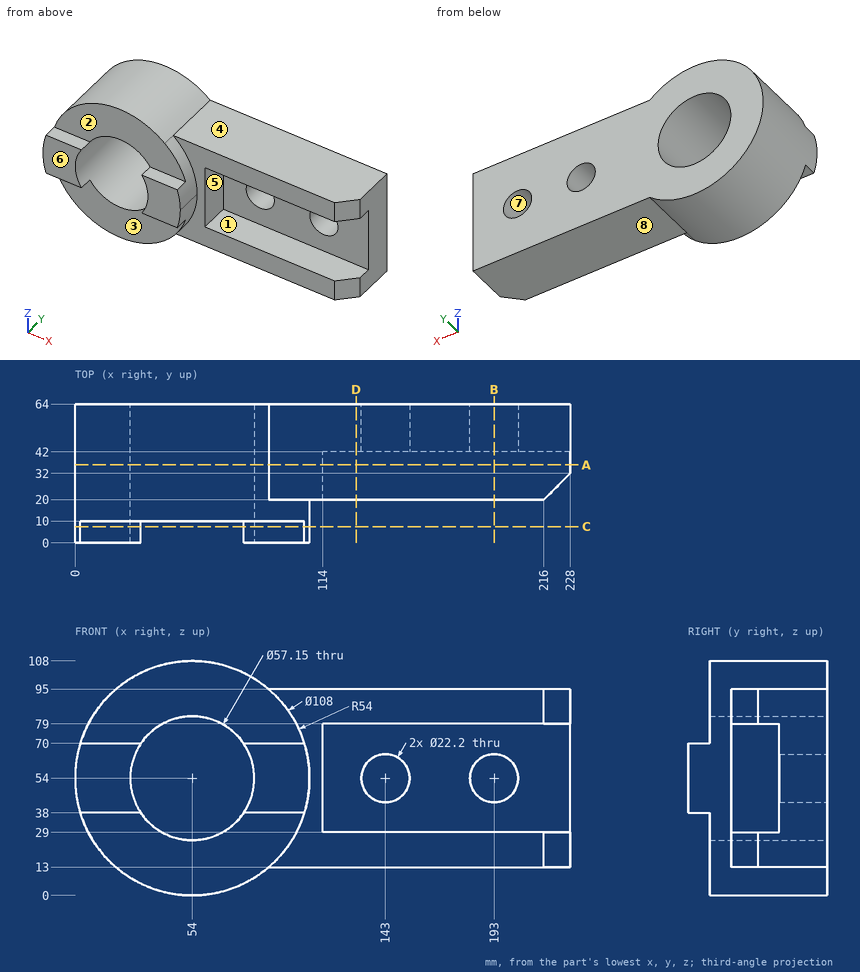
For this review, use the dimensioned drawing (mm, ordinates from the lowest corner) and the shaded views. A direction names the side the tool comes from. Give positions to 0.01 mm unless a question says otherwise; leave off trailing zeros. Loops run counter-clockwise (first coordinate to the right, second up) from the corner with the lowest first, then second, coordinate; pieces in that order, holes last.
Item 1: Take a section at D-D, the plane x = 129.5. State the section outline as (y, z) points.
Item 2: For line 1 along Z through (x, y) = (160, 33.5); line 2 along X through (y, z) = (54, 54) (3 decimals); line 3 along Z through (x, y) = (193, 47), list the stretches that pass through material, from the lowest coordinate up.
Item 3: Tool access review of the marked faces 1, 2, 3 and 4: name each direction out of +Z, -Z, +X, -X, +Y, -Y from which nothing blocks a thin tool from reaching the whole face with its end or side.
Item 4: Take a section at C-C, the plane y = 7.5. State the section outline as (x, z) points (3 decimals).
Item 5: Draft analysis for pull direction Z (two halves, no side actions). For the marked faces 5, 6, 7 and 8, state which applies: +Z half, -Z half, draft (parallel to the pull), parting line (faces both ways), or undercut.
Item 6: Insertion check: pin 1 (24 mm diameter, centred on x = 151, y = 32.5, fed in from -Z); pin 2 (8 mm diameter, centred on x = 112.5, y = 44.5, fed in from +Z); pin 3 (2 mm diameter, centred on y = 26, z = 13.5, fed in from -X). Each pin has a flat end and moves straight along its axis. Give the tip position at first contact, or say it passes through.
Item 7: Take a section at A-A, the plane y = 36. State the section outline as (x, z) points (3 decimals).
Item 8: Take a section at B-B, the plane x = 193. State the section outline as (y, z) points.
Calculated:
1. outline: (20, 13) - (64, 13) - (64, 95) - (20, 95) - (20, 79) - (42, 79) - (42, 29) - (20, 29) - close
2. line 1: z = 13 to 29, 79 to 95
2. line 2: x = 0 to 25.425, 82.575 to 131.9, 154.1 to 181.9, 204.1 to 228
2. line 3: z = 13 to 42.9, 65.1 to 95
3. face 1: +X, -Y
3. face 2: +Z, +X, -X, -Y
3. face 3: -Z, +X, -X, -Y
3. face 4: +Z, +X, +Y, -Y
4. outline: (2.425, 38) - (30.324, 38) arc R28.575 cw to (30.324, 70) - (2.425, 70) arc R54 ccw to start; (77.676, 38) - (105.575, 38) arc R54 ccw to (105.575, 70) - (77.676, 70) arc R28.575 cw to start
5. face 5: undercut
5. face 6: draft
5. face 7: undercut
5. face 8: -Z half
6. pin 1: stops at z = 13
6. pin 2: stops at z = 95
6. pin 3: stops at x = 17.18
7. outline: (89.143, 13) - (228, 13) - (228, 29) - (114, 29) - (114, 79) - (228, 79) - (228, 95) - (89.143, 95) arc R54 ccw (long way) to start; hole circle Ø57.15 at (54, 54)
8. outline: (20, 13) - (64, 13) - (64, 42.9) - (42, 42.9) - (42, 29) - (20, 29) - close; (20, 79) - (42, 79) - (42, 65.1) - (64, 65.1) - (64, 95) - (20, 95) - close
